CAD build for the part. Positions are in the model's coordinates, mm. A direction names the side the tool comes from. Give positions to 0.01 mm unless a question says otherwise; leave off trailing zeros. Answer as CSV lines item,"result".
```python
from build123d import *

# Parameters (mm, degrees)
F1_DEPTH = 1070
F2_R     = 2
F3_R     = 1
F4_DEPTH = 1070


with BuildPart() as f1:
    # F0 (on Top) → F1 (new body)
    with BuildSketch(Plane.XY):
        Polygon((75, 12.5), (0, 12.5), (-75, 12.5), (-75, 2.5), (-70, 2.5), (-70, 0), (-70, -2.5), (-75, -2.5), (-75, -12.5), (0, -12.5), (75, -12.5), (75, -2.5), (70, -2.5), (70, 0), (70, 2.5), (75, 2.5), align=None)
        Polygon((-65, -7.5), (-65, 0), (-65, 7.5), (-36.25, 7.5), (-36.25, 0), (-36.25, -7.5), align=None, mode=Mode.SUBTRACT)
        Polygon((-31.25, -7.5), (-31.25, 0), (-31.25, 7.5), (-2.5, 7.5), (-2.5, 0), (-2.5, -7.5), align=None, mode=Mode.SUBTRACT)
        Polygon((2.5, 0), (2.5, 7.5), (31.25, 7.5), (31.25, 0), (31.25, -7.5), (2.5, -7.5), align=None, mode=Mode.SUBTRACT)
        Polygon((65, 7.5), (65, 0), (65, -7.5), (36.25, -7.5), (36.25, 0), (36.25, 7.5), align=None, mode=Mode.SUBTRACT)
    extrude(amount=F1_DEPTH)

    # F2
    f2_edges = [f1.edges().sort_by_distance(p)[0] for p in [
        (75, -12.5, 535),
        (75, 12.5, 535),
        (-75, -12.5, 535),
        (-75, 12.5, 535),
    ]]
    fillet(f2_edges, radius=F2_R)

    # F3 (on face) → F4 (cut)
    with BuildSketch(Plane.XY.offset(1070)):
        with Locations((-65, 12.5)):
            Circle(F3_R)
        with Locations((-65, -12.5)):
            Circle(F3_R)
        with Locations((-60, 12.5)):
            Circle(F3_R)
        with Locations((-60, -12.5)):
            Circle(F3_R)
        with Locations((-55, 12.5)):
            Circle(F3_R)
        with Locations((-55, -12.5)):
            Circle(F3_R)
        with Locations((-50, 12.5)):
            Circle(F3_R)
        with Locations((-50, -12.5)):
            Circle(F3_R)
        with Locations((-45, 12.5)):
            Circle(F3_R)
        with Locations((-45, -12.5)):
            Circle(F3_R)
        with Locations((-40, 12.5)):
            Circle(F3_R)
        with Locations((-40, -12.5)):
            Circle(F3_R)
        with Locations((-35, 12.5)):
            Circle(F3_R)
        with Locations((-35, -12.5)):
            Circle(F3_R)
        with Locations((-30, 12.5)):
            Circle(F3_R)
        with Locations((-30, -12.5)):
            Circle(F3_R)
        with Locations((-25, 12.5)):
            Circle(F3_R)
        with Locations((-25, -12.5)):
            Circle(F3_R)
        with Locations((-20, 12.5)):
            Circle(F3_R)
        with Locations((-20, -12.5)):
            Circle(F3_R)
        with Locations((-15, 12.5)):
            Circle(F3_R)
        with Locations((-15, -12.5)):
            Circle(F3_R)
        with Locations((-10, 12.5)):
            Circle(F3_R)
        with Locations((-10, -12.5)):
            Circle(F3_R)
        with Locations((-5, 12.5)):
            Circle(F3_R)
        with Locations((-5, -12.5)):
            Circle(F3_R)
        with Locations((0, 12.5)):
            Circle(F3_R)
        with Locations((0, -12.5)):
            Circle(F3_R)
        with Locations((5, 12.5)):
            Circle(F3_R)
        with Locations((5, -12.5)):
            Circle(F3_R)
        with Locations((10, 12.5)):
            Circle(F3_R)
        with Locations((10, -12.5)):
            Circle(F3_R)
        with Locations((15, 12.5)):
            Circle(F3_R)
        with Locations((15, -12.5)):
            Circle(F3_R)
        with Locations((20, 12.5)):
            Circle(F3_R)
        with Locations((20, -12.5)):
            Circle(F3_R)
        with Locations((25, 12.5)):
            Circle(F3_R)
        with Locations((25, -12.5)):
            Circle(F3_R)
        with Locations((30, 12.5)):
            Circle(F3_R)
        with Locations((30, -12.5)):
            Circle(F3_R)
        with Locations((35, 12.5)):
            Circle(F3_R)
        with Locations((35, -12.5)):
            Circle(F3_R)
        with Locations((40, 12.5)):
            Circle(F3_R)
        with Locations((40, -12.5)):
            Circle(F3_R)
        with Locations((45, 12.5)):
            Circle(F3_R)
        with Locations((45, -12.5)):
            Circle(F3_R)
        with Locations((50, 12.5)):
            Circle(F3_R)
        with Locations((50, -12.5)):
            Circle(F3_R)
        with Locations((55, 12.5)):
            Circle(F3_R)
        with Locations((55, -12.5)):
            Circle(F3_R)
        with Locations((60, 12.5)):
            Circle(F3_R)
        with Locations((60, -12.5)):
            Circle(F3_R)
        with Locations((65, 12.5)):
            Circle(F3_R)
        with Locations((65, -12.5)):
            Circle(F3_R)
    extrude(amount=-F4_DEPTH, mode=Mode.SUBTRACT)


solid = f1.part
```
1) Pull direction Y, two halves, no side cores. Call faces 1 (the flat face through (-50, -7.5, 528)), 2 (the flat face through (-1, 0, 1070)): pulls with the +Y half, pulls with the -Y half, needs draft (parallel to the pull), parting line crosses it, or undercut.
Data:
face 1,"undercut"
face 2,"needs draft"
2) Band-saw the part on A-A, the plane z = 780.5. Give the number of separate pieces and of enclosed holes in the cut face, then the cut area to 3 significant figures.
Data:
separate pieces,"1"
enclosed holes,"4"
area,"1,890 mm2"
3) Wall check: line 1 along X through (y, z) = (5.5, 354.5); line 2 along X through (y, z) = (0, 218); line 3 along Y through (x, z) = (-5, 630). Give the ranges that are in metal, low to high. Write a range as [from, to].
Data:
line 1,"x = [-75, -65], [-36.25, -31.25], [-2.5, 2.5], [31.25, 36.25], [65, 75]"
line 2,"x = [-70, -65], [-36.25, -31.25], [-2.5, 2.5], [31.25, 36.25], [65, 70]"
line 3,"y = [-11.5, -7.5], [7.5, 11.5]"
4) Which spindle directions (+Z, -Z, +X, -X, +Y, -Y) get a long thin tool onto all of the face, cutting with end or side? Do faces 3 (the flat face through (-1, 0, 0)), 4 (the flat face through (51, -7.5, 528)). Say none if no direction does.
Data:
face 3,"-Z, +X, -X, +Y, -Y"
face 4,"+Z, -Z"
5) Pin check, flat tip, straight feed: P1, Ø4.5, axis at y = 0, z = 521.5, coming from the -X side. Stop position of the tip, or through.
Data:
P1,"stops at x = -70"
